```python
from build123d import *

# Parameters (mm, degrees)
F2_R     = 1.75
F3_DEPTH = 25


# Not quite as in the source:
# - a fillet or chamfer that OpenCascade refuses, or shapes differently, is made with other operations: its cross-section is extruded or revolved along the edge and cut away or added


with BuildPart() as f1:
    # F0 (on Front) → F1 (revolve)
    with BuildSketch(Plane.XZ):
        Polygon((-4, 0), (0, 0), (0, 10), (-2.5, 10), (-3.1176584307, 7.3764383901), (-3.1176584307, 3.7520567627), (-2.5, 2.8), (-2.5, 0.8), (-4, 0.8), align=None)
    revolve(axis=Axis((0, 0, 5), (0, 0, 1)))

    # F2 (on face) → F3 (cut)
    with BuildSketch(Plane.XY.offset(10)):
        Circle(F2_R)
    extrude(amount=-F3_DEPTH, mode=Mode.SUBTRACT)

    # F4: fillet of radius 1 on 7 edges, made by hand

    # F4_s1 → F4_t2 (revolve)
    with BuildSketch(Plane.XZ):
        with BuildLine():
            ThreePointArc((-2.4996, 2.5034415217), (-2.5408144836, 2.7879202783), (-2.6610688008, 3.0490058884))
            Line((-2.6610688008, 3.0490058884), (-2.5769756809, 3.1035623251))
            ThreePointArc((-2.5769756809, 3.1035623251), (-2.4966090641, 2.9789505293), (-2.4159068801, 2.8545564367))
            Line((-2.4159068801, 2.8545564367), (-2.39976, 2.8))
            ThreePointArc((-2.39976, 2.8), (-2.39976, 2.6517207608), (-2.39936, 2.5034415217))
            Line((-2.39936, 2.5034415217), (-2.4996, 2.5034415217))
        make_face()
    revolve(axis=Axis((0, 0, 2.8), (0, 0, 1)))

    # F4_s3 → F4_t4 (revolve, cut)
    with BuildSketch(Plane.XZ):
        with BuildLine():
            ThreePointArc((-1.7069387157, 10.0004), (-2.3289092353, 9.7839522663), (-2.6821291124, 9.2281351497))
            Line((-2.6821291124, 9.2281351497), (-2.7796481521, 9.251093809))
            ThreePointArc((-2.7796481521, 9.251093809), (-2.6883889182, 9.6369804016), (-2.5975190397, 10.0229586592))
            Line((-2.5975190397, 10.0229586592), (-2.5, 10.1001851443))
            ThreePointArc((-2.5, 10.1001851443), (-2.1034693578, 10.1001851443), (-1.7069387157, 10.1005851443))
            Line((-1.7069387157, 10.1005851443), (-1.7069387157, 10.0004))
        make_face()
    revolve(axis=Axis((0, 0, 10), (0, 0, 1)), mode=Mode.SUBTRACT)

    # F4_s5 → F4_t6 (revolve, cut)
    with BuildSketch(Plane.XZ):
        with BuildLine():
            ThreePointArc((-3.0913827866, 7.489792119), (-3.1113671869, 7.3757078111), (-3.1180584307, 7.2600798179))
            Line((-3.1180584307, 7.2600798179), (-3.2182984307, 7.2600798179))
            ThreePointArc((-3.2182984307, 7.2600798179), (-3.2178984307, 7.318259104), (-3.2178984307, 7.3764383901))
            Line((-3.2178984307, 7.3764383901), (-3.2152308663, 7.3994096202))
            ThreePointArc((-3.2152308663, 7.3994096202), (-3.2018983666, 7.4560406522), (-3.1889552222, 7.5127633491))
            Line((-3.1889552222, 7.5127633491), (-3.0913827866, 7.489792119))
        make_face()
    revolve(axis=Axis((0, 0, 7.3764383901), (0, 0, 1)), mode=Mode.SUBTRACT)

    # F4_s7 → F4_t8 (revolve, cut)
    with BuildSketch(Plane.XZ):
        with BuildLine():
            ThreePointArc((-3.1180584307, 4.048615241), (-3.0768439472, 3.7641364844), (-2.9565896299, 3.5030508742))
            Line((-2.9565896299, 3.5030508742), (-3.0406827498, 3.4484944376))
            ThreePointArc((-3.0406827498, 3.4484944376), (-3.1210493667, 3.5731062334), (-3.2017515506, 3.697500326))
            Line((-3.2017515506, 3.697500326), (-3.2178984307, 3.7520567627))
            ThreePointArc((-3.2178984307, 3.7520567627), (-3.2178984307, 3.9003360018), (-3.2182984307, 4.048615241))
            Line((-3.2182984307, 4.048615241), (-3.1180584307, 4.048615241))
        make_face()
    revolve(axis=Axis((0, 0, 3.7520567627), (0, 0, 1)), mode=Mode.SUBTRACT)


solid = f1.part
```
Read the model definition and answer for the solid it produces. Units are mm, in the model's axes. A direction names the side the tool comes from. Round coordinates to 2 decimals unless told otherwise and drop trailing zeros. Write each loop counter-clockwise with the first axis right and the second up, starting at its lowest first coordinate (ties: lowest second). Pieces come first, ordered by that corner, then holes. Notation, with made-up numbers: (-11.75, 24.25) - (26.25, 24.25) arc R13 cw to (26.25, 34.25) - close; hole circle Ø5 at (-7.75, 6). An arc over 180 degrees is marked (long way). One line per item, written item: value.
Q1. Find section C-C (z = 7). Determine the outline of the cut face in (x, y).
The answers:
outline: circle Ø6.24 at (0, 0); hole circle Ø3.5 at (0, 0)
Q2. For a pull along Z with two mould halves and no side action, classify faces 1 (the cylindrical face through (0.867, 3.905, 0.394)), 2 (the conical face through (2.181, 1.672, 8.944)), 3 (the cylindrical face through (0.54, 2.44, 1.65)), 4 (the flat face through (2, -2, 0.8)) as pulls with the +Z half, pulls with the -Z half, needs draft (parallel to the pull), parting line crosses it, or undercut.
The answers:
face 1: needs draft
face 2: pulls with the +Z half
face 3: undercut
face 4: undercut
Q3. Straight lines are drawn through the part: line 1 (X direction, y = 0, z = 5); line 2 (X direction, y = 0, z = 1). For each, find the intervals that lie inside material, in ascending order. Write a range as from..to.
The answers:
line 1: x = -3.12..-1.75, 1.75..3.12
line 2: x = -2.5..-1.75, 1.75..2.5
Q4. Each of these flat-tipped pins is pushed along its axis until it touches: P1, Ø2, axis at x = -2, z = 4.5, coming from the -Y side; P2, Ø2, axis at x = 0, y = 0, coming from the +Z side; P3, Ø1, axis at x = -3, z = 8.5, coming from the +Y side. Where does it stop, or does it pass through?
The answers:
P1: stops at y = -2.95
P2: passes through
P3: stops at y = 1.41
Q5. Which of the six approach directions +Z, -Z, +X, -X, +Y, -Y give full straight-line access (tool end or side, diameter ignored) to faces 5 (the flat face through (-2, 1, 0)), 6 (the cylindrical face through (-2.974, -0.936, 5.631))?
The answers:
face 5: -Z, +X, -X, +Y, -Y
face 6: +Z
Q6. Find section A-A (y = 0). Determine the outline of the cut face in (x, z), and give its area (3 significant figures).
The answers:
outline: (-4, 0) - (-1.75, 0) - (-1.75, 10) arc R1 ccw to (-2.68, 9.26) - (-3.1, 7.46) arc R1 ccw to (-3.12, 7.29) - (-3.12, 4.02) arc R1 ccw to (-2.97, 3.53) - (-2.65, 3.03) arc R1 cw to (-2.5, 2.53) - (-2.5, 0.8) - (-4, 0.8) - close; (1.75, 0) - (4, 0) - (4, 0.8) - (2.5, 0.8) - (2.5, 2.53) arc R1 cw to (2.65, 3.03) - (2.97, 3.53) arc R1 ccw to (3.12, 4.02) - (3.12, 7.29) arc R1 ccw to (3.1, 7.46) - (2.68, 9.26) arc R1 ccw to (1.75, 10) - close
area: 23.8 mm2
Q7. Find section D-D (y = 3.5). Determine the outline of the cut face in (x, z), and give its area (3 significant figures).
The answers:
outline: (-1.94, 0) - (1.94, 0) - (1.94, 0.8) - (-1.94, 0.8) - close
area: 3.10 mm2
